Autodesk Inventor part; units mm, degrees
ref_plane "YZ Plane" through (0, 0, 0) normal (1, 0, 0) x (0, 1, 0)
ref_plane "XZ Plane" through (0, 0, 0) normal (0, 1, 0) x (-1, 0, 0)
ref_plane "XY Plane" through (0, 0, 0) normal (0, 0, 1) x (1, 0, 0)
sketch "Sketch1" plane through (0, 0, 0) normal (0, 0, 1) x (1, 0, 0)
  line L0 (-66.7657, 11.6667) -> (16.2343, 11.6667)
  line L1 (16.2343, 11.6667) -> (16.2343, -23.3333)
  line L2 (16.2343, -23.3333) -> (-66.7657, -23.3333)
  line L3 (-66.7657, -23.3333) -> (-66.7657, 11.6667)
  point P0 (0, 0)
  dimension "d0" = 35
  dimension "d1" = 83
extrude "Extrusion1" add sketch "Sketch1" along normal blind 1.2
sketch "Sketch2" plane through (0, 0, 1.2) normal (0, 0, 1) x (1, 0, 0)
  line L0 (16.2343, -23.3333) -> (16.2343, 11.6667)
  line L1 (-66.7657, 11.6667) -> (16.2343, 11.6667)
  line L2 (16.2343, 11.6667) -> (16.2343, 9.8667)
  line L3 (16.2343, 9.8667) -> (-66.7657, 9.8667)
  line L4 (-66.7657, 9.8667) -> (-66.7657, 11.6667)
  line L5 (-66.7657, 11.6667) -> (-66.7657, -23.3333)
  line L6 (16.2343, -23.3333) -> (-66.7657, -23.3333)
  line L7 (-66.7657, -23.3333) -> (-66.7657, -21.5333)
  line L8 (-66.7657, -21.5333) -> (16.2343, -21.5333)
  line L9 (16.2343, -21.5333) -> (16.2343, -23.3333)
  line L10 (-66.7657, 9.8667) -> (-65.5657, 9.8667)
  line L11 (-65.5657, 9.8667) -> (-65.5657, -21.5333)
  line L12 (-65.5657, -21.5333) -> (-66.7657, -21.5333)
  line L13 (-66.7657, -21.5333) -> (-66.7657, 9.8667)
  line L14 (16.2343, 9.8667) -> (15.0343, 9.8667)
  line L15 (15.0343, 9.8667) -> (15.0343, -21.5333)
  line L16 (15.0343, -21.5333) -> (16.2343, -21.5333)
  line L17 (16.2343, -21.5333) -> (16.2343, 9.8667)
  line L18 (-66.7657, 11.6667) -> (-65.5657, 11.6667)
  line L19 (-65.5657, 11.6667) -> (-65.5657, -21.5333)
  line L20 (-65.5657, -21.5333) -> (-66.7657, -21.5333)
  line L21 (-66.7657, -21.5333) -> (-66.7657, 11.6667)
  line L22 (-66.7657, 11.6667) -> (16.2343, 11.6667)
  line L23 (16.2343, 11.6667) -> (16.2343, 9.8667)
  line L24 (16.2343, 9.8667) -> (-66.7657, 9.8667)
  line L25 (-66.7657, 9.8667) -> (-66.7657, 11.6667)
  point P0 (0, 0)
  dimension "d4" = 1.8
  dimension "d5" = 1.8
  dimension "d6" = 1.2
  dimension "d7" = 1.2
extrude "Extrusion2" add sketch "Sketch2" along normal blind 30 contours L6 L5 L8 L0 | L8 L15 L3 L0 | L3 L19 L1 L0 | L5 L3 L11 L8 | L4 L1 L19 L3
sketch "Sketch3" plane through (0, 0, 31.2) normal (0, 0, 1) x (1, 0, 0)
  point P0 (0, 0)
sketch "Sketch4" plane through (16.2343, -23.3333, 0) normal (1, 0, 0) x (0, 0, -1)
  line L0 (-1.2, 33.2) -> (-1.2, 1.8)
  line L1 (-1.2, 7.5) -> (-6.2, 7.5)
  line L2 (-6.2, 7.5) -> (-6.2, 27.5)
  line L3 (-6.2, 27.5) -> (-1.2, 27.5)
  line L4 (-1.2, 27.5) -> (-1.2, 7.5)
  line L5 (-1.2, 1.8) -> (-31.2, 1.8)
  line L6 (-1.2, 33.2) -> (-31.2, 33.2)
  line L7 (-6.2, 7.5) -> (0, 7.5)
  line L8 (0, 7.5) -> (0, 27.5)
  line L9 (0, 27.5) -> (-6.2, 27.5)
  line L10 (-6.2, 27.5) -> (-6.2, 7.5)
  line L11 (0, 35) -> (0, 0)
  point P0 (0, 23.3333)
  dimension "d10" = 20
  dimension "d11" = 5
  dimension "d12" = 5.7
  dimension "d13" = 5.7
extrude "Extrusion3" cut sketch "Sketch4" against normal blind 10
fillet "Fillet1" radius 2 8 edges at (-66.7657, 11.6667, 15.6) (-65.5657, 9.8667, 16.2) (-66.7657, -23.3333, 15.6) (-65.5657, -21.5333, 16.2) (15.0343, 9.8667, 16.2) (16.2343, 11.6667, 15.6) (16.2343, -23.3333, 15.6) (15.0343, -21.5333, 16.2)
sketch "Sketch5" plane through (0, 0, 1.2) normal (0, 0, 1) x (1, 0, 0)
  circle A0 centre (10.0343, 6.6667) radius 1.5
  circle A1 centre (10.0343, -18.3333) radius 1.5
  line L0 (15.0343, 7.8667) -> (15.0343, -19.5333)
  line L1 (13.0343, -21.5333) -> (-63.5657, -21.5333)
  line L2 (-63.5657, 9.8667) -> (13.0343, 9.8667)
  point P0 (0, 0)
  dimension "d17" = 3
  dimension "d18" = 3
  dimension "d19" = 25
  dimension "d20" = 5
  dimension "d21" = 5
  dimension "d22" = 3.2
  dimension "d23" = 3.2
extrude "Extrusion4" add sketch "Sketch5" along normal blind 5
sketch "Sketch6" plane through (0, 0, 1.2) normal (0, 0, 1) x (1, 0, 0)
  circle A0 centre (-41.9656, -18.3962) radius 1.5
  circle A1 centre (-41.9656, 6.6038) radius 1.5
  circle A2 centre (10.0343, 6.6667) radius 1.5
  circle A3 centre (10.0343, -18.3333) radius 1.5
  point P0 (0, 0)
  dimension "d26" = 3
  dimension "d27" = 3
  dimension "d28" = 25
  dimension "d29" = 52
  dimension "d30" = 52
extrude "Extrusion5" add sketch "Sketch6" along normal blind 5 contours A0 | A1
sketch "Sketch7" plane through (-41.9656, 6.6038, 6.2) normal (0, 0, 1) x (1, 0, 0)
  point P0 (41.9656, -6.6038)
sketch "Sketch8" plane through (0, 0, 1.2) normal (0, 0, 1) x (1, 0, 0)
  circle A0 centre (-41.9656, -18.3962) radius 1.5
  circle A1 centre (-41.9656, -18.3962) radius 3
  circle A2 centre (-41.9656, 6.6038) radius 1.5
  circle A3 centre (-41.9656, 6.6038) radius 3
  circle A4 centre (10.0343, -18.3333) radius 1.5
  circle A5 centre (10.0343, -18.3333) radius 3
  circle A6 centre (10.0343, 6.6667) radius 1.5
  circle A7 centre (10.0343, 6.6667) radius 3
  point P0 (0, 0)
  dimension "d33" = 6
  dimension "d34" = 6
  dimension "d35" = 6
  dimension "d36" = 6
extrude "Extrusion6" add sketch "Sketch8" along normal blind 5
sketch "Sketch9" plane through (0, 0, 1.2) normal (0, 0, 1) x (1, 0, 0)
  arc A0 (8.376, -15.8333) -> (11.6926, -15.8333) centre (10.0343, -18.3333) ccw
  circle A1 centre (10.0343, -18.3333) radius 3
  arc A2 (11.6926, 4.1667) -> (8.376, 4.1667) centre (10.0343, 6.6667) ccw
  circle A3 centre (10.0343, 6.6667) radius 3
  point P0 (0, 0)
  dimension "d39" = 6
  dimension "d40" = 6
extrude "Extrusion7" add sketch "Sketch9" against normal blind 1.2
sketch "Sketch10" plane through (-41.9656, -18.3962, 6.2) normal (0, 0, 1) x (1, 0, 0)
  circle A0 centre (0, 0) radius 3
  circle A1 centre (0, 0) radius 1.5
  circle A2 centre (0, 25) radius 3
  circle A3 centre (0, 25) radius 1.5
  circle A4 centre (52, 0.0629) radius 3
  circle A5 centre (52, 0.0629) radius 1.5
  circle A6 centre (52, 25.0629) radius 3
  circle A7 centre (52, 25.0629) radius 1.5
  point P0 (41.9656, 18.3962)
  dimension "d43" = 3
  dimension "d44" = 3
  dimension "d45" = 3
  dimension "d46" = 3
extrude "Extrusion8" cut sketch "Sketch10" against normal blind 4 contours A1 | A3 | A5 | A7
thread "Thread1"
thread "Thread2"
thread "Thread3"
thread "Thread4"
sketch "Sketch11" plane through (0, 0, 31.2) normal (0, 0, 1) x (1, 0, 0)
  arc A0 (-64.7657, 11.6667) -> (-66.7657, 9.6667) centre (-64.7657, 9.6667) ccw
  line L0 (-66.7657, 9.6667) -> (16.2343, 9.6667)
  line L1 (16.2343, 9.6667) -> (16.2343, 14.6667)
  line L2 (16.2343, 14.6667) -> (-66.7657, 14.6667)
  line L3 (-66.7657, 14.6667) -> (-66.7657, 9.6667)
  line L4 (16.2343, -21.3333) -> (-66.7657, -21.3333)
  line L5 (-66.7657, -21.3333) -> (-66.7657, -26.3333)
  line L6 (-66.7657, -26.3333) -> (16.2343, -26.3333)
  line L7 (16.2343, -26.3333) -> (16.2343, -21.3333)
  point P0 (0, 0)
  dimension "d57" = 5
  dimension "d58" = 5
  dimension "d59" = 83
extrude "Extrusion9" add sketch "Sketch11" against normal blind 31.2
fillet "Fillet2" radius 2 4 edges at (16.2343, -26.3333, 15.6) (16.2343, 14.6667, 15.6) (-66.7657, 14.6667, 15.6) (-66.7657, -26.3333, 15.6)
sketch "Sketch12" plane through (0, 0, 31.2) normal (0, 0, 1) x (1, 0, 0)
  line L0 (14.2343, -26.3333) -> (-64.7657, -26.3333)
  line L1 (8.2343, -26.3333) -> (-58.7657, -26.3333)
  line L2 (-58.7657, -26.3333) -> (-58.7657, -23.1333)
  line L3 (-58.7657, -23.1333) -> (8.2343, -23.1333)
  line L4 (8.2343, -23.1333) -> (8.2343, -26.3333)
  line L5 (-64.7657, 14.6667) -> (14.2343, 14.6667)
  line L6 (8.2343, 14.6667) -> (-58.7657, 14.6667)
  line L7 (-58.7657, 14.6667) -> (-58.7657, 11.4667)
  line L8 (-58.7657, 11.4667) -> (8.2343, 11.4667)
  line L9 (8.2343, 11.4667) -> (8.2343, 14.6667)
  line L10 (16.2343, -24.3333) -> (16.2343, 12.6667)
  line L11 (-66.7657, 12.6667) -> (-66.7657, -24.3333)
  line L12 (13.9061, -21.3333) -> (-64.4375, -21.3333)
  line L13 (10.0343, 9.6667) -> (-64.4375, 9.6667)
  point P0 (0, 0)
  dimension "d63" = 8
  dimension "d64" = 8
  dimension "d65" = 1.8
  dimension "d66" = 1.8
extrude "Extrusion10" cut sketch "Sketch12" against normal blind 31.2
fillet "Fillet3" radius 2 4 edges at (8.2343, -26.3333, 15.6) (-58.7657, -26.3333, 15.6) (8.2343, 14.6667, 15.6) (-58.7657, 14.6667, 15.6)
sketch "Sketch13" plane through (0, 0, 31.2) normal (0, 0, 1) x (1, 0, 0)
  line L0 (14.2343, -26.3333) -> (10.2343, -26.3333)
  circle A0 centre (12.2343, -23.9333) radius 1.5
  circle A1 centre (-62.7657, -23.9333) radius 1.5
  line L1 (-64.7657, -26.3333) -> (-60.7657, -26.3333)
  circle A2 centre (12.2343, 12.2667) radius 1.5
  circle A3 centre (-62.7657, 12.2667) radius 1.5
  line L2 (-66.7657, 12.6667) -> (-66.7657, -24.3333)
  line L3 (-60.7657, 14.6667) -> (-64.7657, 14.6667)
  line L4 (16.2343, -24.3333) -> (16.2343, 12.6667)
  line L5 (14.2343, 14.6667) -> (10.2343, 14.6667)
  line L6 (8.2343, -23.1333) -> (8.2343, -24.3333)
  point P0 (0, 0)
  dimension "d70" = 2.4
  dimension "d71" = 3
  dimension "d72" = 3
  dimension "d73" = 2.4
  dimension "d74" = 3
  dimension "d75" = 3
  dimension "d76" = 4
  dimension "d77" = 4
  dimension "d78" = 2.4
  dimension "d79" = 4
  dimension "d80" = 2.4
  dimension "d81" = 4
hole "Hole1" at (12.2343, -23.9333, 31.2) at (12.2343, 12.2667, 31.2) at (-62.7657, -23.9333, 31.2) at (-62.7657, 12.2667, 31.2) direction (0, 0, -1) diameter 3 depth 5 tip angle 118
properties part number "Case Bottom"
Work out the finished part from the listing and answer in its coordinate system (mm). A direction names the side the tool comes from. Round coordinates to 2 decimals unless told otherwise and drop trailing zeros. Write each loop counter-clockwise with the first axis right and the second up, starting at its lowest first coordinate (ties: lowest second). Pieces come first, ordered by that corner, then holes.
1) A cutting plane is placed at B-B (z = 15.5). Give the vertices of the cut face in (x, y).
2) A cutting plane is placed at C-C (x = -17). Give the vertices of the cut face in (y, z).
3) Straight lines are drawn through the part: line 1 (X direction, y = 1.5, z = 23.5); line 2 (X direction, y = 11.5, z = 3); line 3 (Y direction, x = -8, z = 27). For each, find the intervals that lie inside material, in ascending order.
4) A tool of negligible diameter and unlimited length cuts with its end or side. For faces 4 (the cylindrical face through (8.805, 14.065, 15.382)), 5 (the flat face through (-63, -26.333, 16)), 6 (the flat face through (9, 8, 6.2)), 7 (the flat face through (-26, -23.133, 16)), from which of +Z, -Z, +X, -X, +Y, -Y can it reach the whole face along a straight path? Write none if from no direction.
5) The mould has two halves that part along X. Classify faces 1 (the flat face through (-42, -18, 2.2)), 2 (the cylindrical face through (-64.253, -23.738, 28.665)), 3 (the flat face through (16, 4.167, 2)): pulls with the +X half, pulls with the -X half, needs draft (parallel to the pull), parting line crosses it, or undercut.
6) A cutting plane is placed at A-A (y = -7). Give the vertices of the cut face in (x, z), plus the area to 3 significant figures.
7) Given pin 1 Ø3.5 at (x, y) = (12.23, 12.27) entering from +Z; pin 2 Ø1.8 at (x, y) = (-41.97, 6.6) entering from +Z; pin 3 Ø1.3 at (x, z) = (7, 0.5) entering from -Y; pin 4 Ø3 at (x, z) = (-8.5, 25) entering from +Y, each flat-ended and moving along its own axis, determine where each tip first touches the part or whether it passes through.
Completed:
1. outline: (-66.77, -24.33) arc R2 ccw to (-64.77, -26.33) - (-60.77, -26.33) arc R2 ccw to (-58.77, -24.33) - (-58.77, -23.13) - (8.23, -23.13) - (8.23, -24.33) arc R2 ccw to (10.23, -26.33) - (14.23, -26.33) arc R2 ccw to (16.23, -24.33) - (16.23, 12.67) arc R2 ccw to (14.23, 14.67) - (10.23, 14.67) arc R2 ccw to (8.23, 12.67) - (8.23, 11.47) - (-58.77, 11.47) - (-58.77, 12.67) arc R2 ccw to (-60.77, 14.67) - (-64.77, 14.67) arc R2 ccw to (-66.77, 12.67) - close; hole (-65.57, -19.53) arc R2 ccw to (-64.44, -21.33) - (13.91, -21.33) arc R2 ccw to (15.03, -19.53) - (15.03, 7.87) arc R2 ccw to (13.91, 9.67) - (-64.44, 9.67) arc R2 ccw to (-65.57, 7.87) - close
2. outline: (-23.13, 0) - (11.47, 0) - (11.47, 31.2) - (9.67, 31.2) - (9.67, 1.2) - (-21.33, 1.2) - (-21.33, 31.2) - (-23.13, 31.2) - close
3. line 1: x = -66.77 to -65.57, 15.03 to 16.23
3. line 2: x = -66.77 to -58.77, 8.23 to 16.23
3. line 3: y = -23.13 to -21.33, 9.67 to 11.47
4. face 4: +Z, -Z, +Y
4. face 5: +Z, -Z, +X, -X, -Y
4. face 6: +Z
4. face 7: +Z, -Z, -Y
5. face 1: undercut
5. face 2: undercut
5. face 3: needs draft
6. outline: (-66.77, 0) - (6.23, 0) - (6.23, 1.2) - (-65.57, 1.2) - (-65.57, 31.2) - (-66.77, 31.2) - close; (15.03, 6.2) - (16.23, 6.2) - (16.23, 31.2) - (15.03, 31.2) - close
6. area: 154 mm2
7. pin 1: stops at z = 31.2
7. pin 2: stops at z = 2.2
7. pin 3: stops at y = -23.13
7. pin 4: stops at y = 11.47
